Autodesk Inventor part; units mm, degrees
ref_plane "YZ Plane" through (0, 0, 0) normal (1, 0, 0) x (0, 1, 0)
ref_plane "XZ Plane" through (0, 0, 0) normal (0, 1, 0) x (-1, 0, 0)
ref_plane "XY Plane" through (0, 0, 0) normal (0, 0, 1) x (1, 0, 0)
sketch "Sketch1" plane through (0, 0, 0) normal (0, 0, 1) x (1, 0, 0)
  line L0 (-12.7, -20.6375) -> (12.7, -20.6375)
  line L1 (12.7, -20.6375) -> (12.7, 20.6375) construction
  line L2 (12.7, 20.6375) -> (-12.7, 20.6375) construction
  line L3 (-12.7, 20.6375) -> (-12.7, -20.6375) construction
  line L4 (-12.7, -20.6375) -> (12.7, 20.6375) construction
  line L5 (12.7, -20.6375) -> (-12.7, 20.6375) construction
  circle A0 centre (0, 11.1125) radius 2.54
  circle A1 centre (0, -1.5875) radius 2.54 construction
  circle A2 centre (0, -14.2875) radius 2.54
  circle A3 centre (-4.7625, 31.75) radius 9.525 construction
  circle A4 centre (-4.7625, 31.75) radius 2.4892
  arc A5 (0.1258, 35.803) -> (-11.0533, 32.6149) centre (-4.7625, 31.75) ccw
  line L6 (-12.7, 20.6375) -> (-11.0533, 32.6149)
  line L7 (12.7, 20.6375) -> (0.1258, 35.803)
  line L8 (-12.7, 20.6375) -> (-11.1125, 20.6375) construction
  line L9 (-11.1125, 20.6375) -> (-11.1125, -20.6375)
  line L10 (11.1125, -20.6375) -> (11.1125, 20.6375)
  line L11 (12.7, 20.6375) -> (11.1125, 20.6375) construction
  line L12 (-12.7, 20.6375) -> (-12.7, 17.4625)
  line L13 (-11.1125, 17.4625) -> (-12.7, 17.4625)
  line L14 (12.7, 20.6375) -> (12.7, 17.4625)
  line L15 (12.7, 17.4625) -> (11.1125, 17.4625)
  point P0 (0, 0)
  point P1 (0, 0)
  dimension "d0" = 25.4
  dimension "d2" = 5.08
  dimension "d3" = 9.525
  dimension "d6" = 12.7
  dimension "d11" = 6.35
  dimension "d12" = 19.05
  dimension "d13" = 4.9784
  dimension "d14" = 11.1125
  dimension "d15" = 4.7625
  dimension "d27" = 1.5875
  dimension "d28" = 1.5875
  dimension "d32" = 3.175
  dimension "d45" = 12.7
extrude "Extrusion1" add sketch "Sketch1" along normal mid plane 50.8
sketch "Sketch3" plane through (-11.1125, -20.6375, 25.4) normal (-1, 0, 0) x (0, 0, 1)
  line L0 (-50.8, 0) -> (0, 0)
  line L1 (0, 38.1) -> (0, 0)
  line L2 (-50.8, 0) -> (-50.8, 38.1)
  line L3 (-49.2125, 41.275) -> (-1.5875, 41.275)
  line L4 (-1.5875, 41.275) -> (-1.5875, 0)
  line L5 (-1.5875, 0) -> (-49.2125, 0)
  line L6 (-49.2125, 0) -> (-49.2125, 41.275)
  line L7 (-49.2125, 41.275) -> (-1.5875, 0) construction
  line L8 (-1.5875, 41.275) -> (-49.2125, 0) construction
  line L9 (-50.8, 38.1) -> (0, 38.1)
  point P0 (-25.4, 20.6375)
  point P1 (-49.2125, 38.1)
  point P2 (-1.5875, 38.1)
  dimension "d29" = 1.5875
extrude "Extrusion3" cut sketch "Sketch3" against normal through all contours L2 L9 L6 L0 | L4 L9 L1 L0
sketch "Sketch2" plane through (0, 0, 25.4) normal (0, 0, 1) x (1, 0, 0)
  circle A0 centre (-4.7625, 31.75) radius 2.4892
  circle A1 centre (-4.7625, 31.75) radius 10.3188
  point P0 (0, 0)
  dimension "d19" = 20.6375
extrude "Extrusion2" cut sketch "Sketch2" against normal blind 5.5563
mirror "Mirror1" about plane through (0, 0, 0) normal (0, 0, 1) of "Extrusion2"
fillet "Fillet1" radius 3.175 3 edges at (5.3172, 29.5418, 22.6219) (5.3172, 29.5418, -22.6219) (12.7, 20.6375, 0)
fillet "Fillet1" radius 2.286 2 edges at (-12.1611, 24.5572, -22.6219) (-12.1611, 24.5572, 22.6219)
thread "Thread1"
thread "Thread2"
thread "Thread3"
thread "Thread4"
sketch "Sketch4" plane through (-11.1125, -20.6375, -23.8125) normal (0, -1, 0) x (1, 0, 0)
  line L0 (0, 0) -> (22.225, 0)
  line L1 (22.225, 0) -> (22.225, 47.625)
  line L2 (22.225, 47.625) -> (0, 47.625)
  line L3 (0, 0) -> (0, 47.625)
  line L4 (19.05, 41.275) -> (3.175, 41.275)
  line L5 (3.175, 41.275) -> (3.175, 6.35)
  line L6 (3.175, 6.35) -> (19.05, 6.35)
  line L7 (19.05, 6.35) -> (19.05, 41.275)
  point P0 (11.1125, 23.8125)
  dimension "d37" = 3.175
  dimension "d38" = 3.175
  dimension "d39" = 6.35
  dimension "d40" = 6.35
extrude "Extrusion4" cut sketch "Sketch4" against normal up to surface (38.1 mm away) contours L7 L6 L5 L4
fillet "Fillet2" radius 3.175 4 edges at (-7.9375, -1.5875, 17.4625) (7.9375, -1.5875, 17.4625) (7.9375, -1.5875, -17.4625) (-7.9375, -1.5875, -17.4625)
equation "\"d28\" = d27"
equation "\"d38\" = d37"
equation "\"d40\" = d39"
properties part number "F4C9-200-001 Top Bearing Block" material "Aluminum 6061"
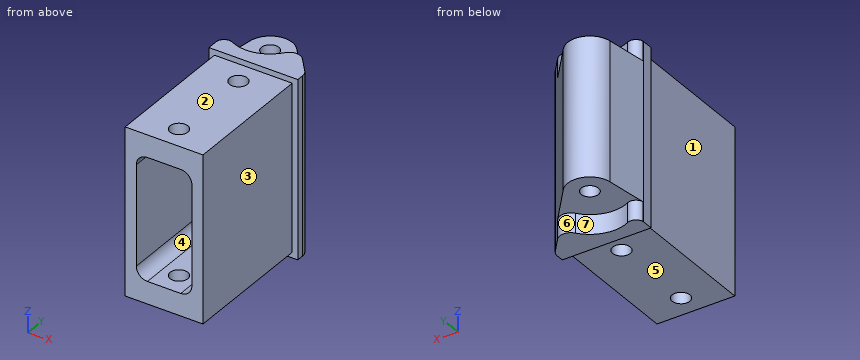
Design review of the part built by this model. Coordinates are the model's own, in mm. Face numbers are marked on the shaded views. A direction names the side the tool comes from. Round coordinates to 2 decimals unless told otherwise and drop trailing zeros. One line per item, written item: value. Start each with the question number.
1) Insertion check: pin 1 Ø6 at (x, y) = (-4.5, -4.5) entering from -Z; pin 2 Ø5 at (x, y) = (-0.5, 3.5) entering from +Z; pin 3 Ø19 at (y, z) = (0, 9.5) entering from +X. Each pin has a flat end and moves straight along its axis. Give the tip position at first contact, or say it passes through.
2) Consider section A-A on z = -18.5. Give the number of separate pieces and of enclosed holes in the cut face, then the cut area to 3 significant figures.
3) Draft analysis for pull direction X (two halves, no side actions). For the marked faces 5, 6 and 7, state which applies: +X half, -X half, draft (parallel to the pull), parting line (faces both ways), or undercut.
4) For the marked faces 1, 2, 3 and 4, list the 3-axis set-ups (+Z, -Z, +X, -X, +Y, -Y) from which the entire face can be reached by the end or side of a thin tool; tool diameter is ignored.
5) To check wall thickness, follow L1, parallel to X at y = 4, z = -7; L2, parallel to Z at x = 5, y = -13.5; L3, parallel to Y at x = 0, z = 20.25. State the ranges of each line that lie inside material, in increasing order. Write a range as from..to.
Reported:
1. pin 1: stops at z = -23.81
1. pin 2: stops at z = 23.81
1. pin 3: stops at x = 11.11
2. separate pieces: 1
2. enclosed holes: 3
2. area: 1,160 mm^2
3. face 5: draft
3. face 6: parting line
3. face 7: undercut
4. face 1: +Z, -Z, -X, -Y
4. face 2: +Z, +X, -X, -Y
4. face 3: +Z, -Z, +X, -Y
4. face 4: -Y
5. L1: x = -11.11..-7.94, 7.94..11.11
5. L2: z = -23.81..-17.45, 17.45..23.81
5. L3: y = -20.64..-16.83, -11.75..8.57, 13.65..22.6
